The listing builds one solid part. Answer for the finished solid, in the listing's coordinates (mm). Face numbers are marked on the shaded views. A direction names the side the tool comes from. Give positions to 0.01 mm unless a question says otherwise; leave off trailing zeros. Write each loop counter-clockwise with the first axis right and the second up, starting at its lowest first coordinate (ties: lowest second). Pieces come first, ordered by that corner, then holes.
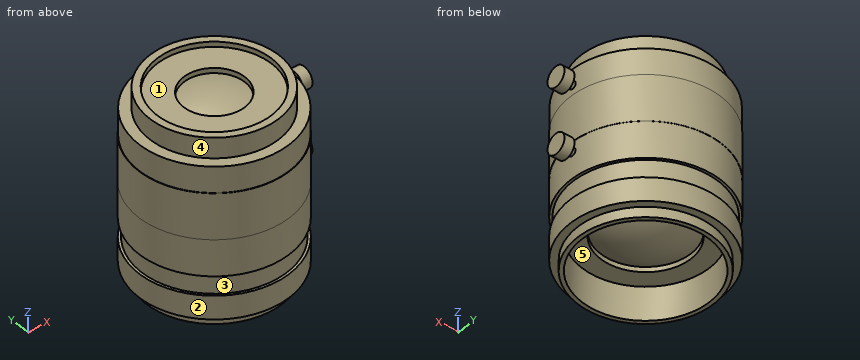
```python
from build123d import *

# Parameters (mm, degrees)
SKETCH1_R       = 13.3
SKETCH1_R_2     = 12.5
EXTRUDE1_DEPTH  = 2
SKETCH2_R       = 14.75
SKETCH2_R_2     = 12.5
EXTRUDE2_DEPTH  = 4.6
SKETCH3_R       = 14.25
EXTRUDE3_DEPTH  = 3.75
SKETCH4_R       = 14.75
EXTRUDE4_DEPTH  = 7.1
SKETCH5_R       = 14.78
EXTRUDE5_DEPTH  = 9
SKETCH6_R       = 14.7
EXTRUDE6_DEPTH  = 5.1
SKETCH7_R       = 12.65
EXTRUDE7_DEPTH  = 4
SKETCH8_R       = 11.25
EXTRUDE8_DEPTH  = 1
SKETCH9_R       = 8.875
EXTRUDE9_DEPTH  = 1
SKETCH10_R      = 6
EXTRUDE10_DEPTH = 1
SKETCH11_R      = 0.75
EXTRUDE11_DEPTH = 16
SKETCH12_R      = 2
EXTRUDE12_DEPTH = 2


# Read off the part's stored shape, not the designer's step: Dome1, Dome2
with BuildPart() as part:
    # Sketch1 → Extrude1 (new body)
    with BuildSketch(Plane.XY):
        Circle(SKETCH1_R)
        Circle(SKETCH1_R_2, mode=Mode.SUBTRACT)
    extrude(amount=EXTRUDE1_DEPTH)

    # Sketch2 → Extrude2 (add)
    with BuildSketch(Plane.XY.offset(2)):
        Circle(SKETCH2_R)
        Circle(SKETCH2_R_2, mode=Mode.SUBTRACT)
    extrude(amount=EXTRUDE2_DEPTH)

    # Sketch3 → Extrude3 (add)
    with BuildSketch(Plane.XY.offset(6.6)):
        Circle(SKETCH3_R)
    extrude(amount=EXTRUDE3_DEPTH)

    # Sketch4 → Extrude4 (add)
    with BuildSketch(Plane.XY.offset(10.35)):
        Circle(SKETCH4_R)
    extrude(amount=EXTRUDE4_DEPTH)

    # Sketch5 → Extrude5 (add)
    with BuildSketch(Plane.XY.offset(17.45)):
        Circle(SKETCH5_R)
    extrude(amount=EXTRUDE5_DEPTH)

    # Sketch6 → Extrude6 (add)
    with BuildSketch(Plane.XY.offset(26.45)):
        Circle(SKETCH6_R)
    extrude(amount=EXTRUDE6_DEPTH)

    # Sketch7 → Extrude7 (add)
    with BuildSketch(Plane.XY.offset(31.55)):
        Circle(SKETCH7_R)
    extrude(amount=EXTRUDE7_DEPTH)

    # Sketch8 → Extrude8 (cut)
    with BuildSketch(Plane.XY.offset(35.55)):
        Circle(SKETCH8_R)
    extrude(amount=-EXTRUDE8_DEPTH, mode=Mode.SUBTRACT)

    # Sketch9 → Extrude9 (cut)
    with BuildSketch(Plane(origin=(0, 0, 6.6), x_dir=(-1, 0, 0), z_dir=(0, 0, -1))):
        Circle(SKETCH9_R)
    extrude(amount=-EXTRUDE9_DEPTH, mode=Mode.SUBTRACT)

    # Dome1 outline → Dome1 (revolve)
    with BuildSketch(Plane.XZ):
        with BuildLine():
            Line((0, 7.600000009), (0, 4.6))
            ThreePointArc((0, 4.6), (4.684165488, 5.370281289), (8.875000012, 7.600000009))
            Line((8.875000012, 7.600000009), (0, 7.600000009))
        make_face()
    revolve(axis=Axis((0, 0, 0), (0, 0, 1)))

    # Sketch10 → Extrude10 (cut)
    with BuildSketch(Plane.XY.offset(34.55)):
        Circle(SKETCH10_R)
    extrude(amount=-EXTRUDE10_DEPTH, mode=Mode.SUBTRACT)

    # Dome2 outline → Dome2 (revolve)
    with BuildSketch(Plane.XZ):
        with BuildLine():
            Line((0, 33.55), (6.000000017, 33.549999994))
            ThreePointArc((6.000000017, 33.549999994), (3.041381274, 34.298287589), (0, 34.55))
            Line((0, 34.55), (0, 33.55))
        make_face()
    revolve(axis=Axis((0, 0, 0), (0, 0, 1)))

    # Sketch11 → Extrude11 (add)
    with BuildSketch(Plane(origin=(0, 0, 0), x_dir=(0, 0, -1), z_dir=(1, 0, 0))):
        with Locations((-28.45, 0)):
            Circle(SKETCH11_R)
        with Locations((-15.45, 0)):
            Circle(SKETCH11_R)
    extrude(amount=EXTRUDE11_DEPTH)

    # Sketch12 → Extrude12 (add)
    with BuildSketch(Plane(origin=(16, 0, 0), x_dir=(0, 0, -1), z_dir=(1, 0, 0))):
        with Locations((-28.45, 0)):
            Circle(SKETCH12_R)
        with Locations((-15.45, 0)):
            Circle(SKETCH12_R)
    extrude(amount=EXTRUDE12_DEPTH)


solid = part.part
```
Item 1: A cutting plane is placed at B-B, the plane y = 1.5. Count the separate pieces of the cut face and the enclosed holes in it, plus the area to 3 significant figures.
Conclusion:
separate pieces: 3
enclosed holes: 0
area: 854 mm2
Item 2: Consider probe 1 along Y at (x, z) = (0, 34.95); probe 2 along Y at (x, z) = (0, 7) (3 decimals); probe 3 along Z at (x, y) = (6.5, -9.5). Determine where each line is inside the solid, lowest interval first.
Conclusion:
probe 1: y = -12.65 to -11.25, 11.25 to 12.65
probe 2: y = -14.25 to -8.875, -8.028 to 8.028, 8.875 to 14.25
probe 3: z = 6.6 to 35.55
Item 3: Which of the six approach directions +Z, -Z, +X, -X, +Y, -Y give full straight-line access (tool end or side, diameter ignored) to the marked faces 3, 4 and 5?
Conclusion:
face 3: none
face 4: +Z
face 5: -Z
Item 4: A cutting plane is placed at A-A, the plane z = 28.45. Give the vertices of the cut face in (x, y), plus the area to 3 significant figures.
Conclusion:
outline: (14.68, -0.75) - (16, -0.75) - (16, -2) - (18, -2) - (18, 2) - (16, 2) - (16, 0.75) - (14.68, 0.75) arc R14.7 ccw (long way) to start
area: 689 mm2
Item 5: Each of these flat-tipped pins is pushed along its axis until it touches: P1, Ø10, axis at y = 6, z = 14.5, coming from the -X side; P2, Ø2, axis at x = -8.5, z = 31.5, coming from the -Y side; P3, Ø7.5, axis at x = 4, y = 3, coming from the -Z side. Where does it stop, or does it pass through?
Conclusion:
P1: stops at x = -14.72
P2: stops at y = -12.64
P3: stops at z = 4.65
Item 6: A cutting plane is placed at D-D, the plane z = 23. Give the vertices of the cut face in (x, y).
Conclusion:
outline: circle Ø29.56 at (0, 0)
Item 7: Determine the mould class of the marked faces 1 and 2 for opening direction Y: pulls with the +Y half, pulls with the -Y half, needs draft (parallel to the pull), parting line crosses it, or undercut.
Conclusion:
face 1: undercut
face 2: parting line crosses it
